Work out the finished part from the listing and answer in its coordinate system (mm). A direction names the side the tool comes from. Coordinates: 2 decimals unless noted, no trailing zeros. Order: outer loops, then holes, each group sorted by start corner. A loop starts at its lowest first (then second) coordinate and runs counter-clockwise, first axis right, second up.
1. Determine the mould class of faces 6 (the cylindrical face through (137.58, 20.95, -2.54)), 7 (the flat face through (-27.1, -18.5, 9.9)), 8 (the cylindrical face through (-1.302, -18.451, 27.915)), 9 (the cylindrical face through (-171.285, -22.813, 4.374)) for opening direction X: +X half, -X half, draft (parallel to the pull), parting line (faces both ways), or undercut.
2. The part is cut by section B-B, the plane z = 15. Give the vertices of the cut face in (x, y), then the cut area to 3 significant figures.
3. A tool of negligible diameter and unlimited length cuts with its end or side. For faces 1 (the flat face through (-7, -22, 9)), 2 (the flat face through (5, 0, 0)), 3 (the cylindrical face through (-174.519, -0.35, 6.433)), 4 (the flat face through (-7, -15, 9)), 5 (the flat face through (7, 22, 9)), from which of +Z, -Z, +X, -X, +Y, -Y can it reach the whole face along a straight path? Write none if from no direction.
4. Flat-ended cylindrical pins translate along their axes: pin 1 Ø12 at (y, z) = (-1, 21.5) entering from +X; pin 2 Ø17.5 at (x, z) = (-5.5, 17.5) entering from +Y; pin 3 Ø5 at (y, z) = (8, 27) entering from -X. Find the tip coordinate at first contact, or state that the pin passes through.
5. The part is cut by section D-D, the plane x = 49. Give the vertices of the cut face in (y, z).
6. Find the intervals of material crossed by probe 1 along Y at (x, z) = (1, 6); probe 2 along Z at (x, y) = (0, -20); probe 3 along Z at (x, y) = (-79, 17.5), in increasing order.
7. The part is cut by section C-C, the plane y = 8.5. Give the vertices of the cut face in (x, z), then the cut area to 3 significant figures.
8. The part is cut by section A-A, the plane x = 0. Give the vertices of the cut face in (y, z).
```python
from build123d import *

# Parameters (mm, degrees)
F0_R     = 10
F1_DEPTH = 25
F2_W     = 30
F2_H     = 40.766016
F2_W_2   = 3
F3_DEPTH = 40
F5_DEPTH = 40.001


with BuildPart() as f1:
    # F0 (on Front) → F1 (new body, symmetric)
    with BuildSketch(Plane.XZ):
        with BuildLine():
            Line((-31.201941, 0), (-147.458184, 0))
            ThreePointArc((-147.458184, 0), (-174.873856, 6.613726), (-196.258555, 25))
            Line((-196.258555, 25), (-197.63568, 23.332754))
            ThreePointArc((-197.63568, 23.332754), (-175.850829, 3.315154), (-147.458184, -5))
            Line((-147.458184, -5), (153.741445, -5))
            Line((153.741445, -5), (153.741445, 0))
            Line((153.741445, 0), (31.201941, 0))
            Line((31.201941, 0), (-31.201941, 0))
        make_face()
        with BuildLine():
            Line((-23.096988, 19.567086), (-31.201941, 0))
            Line((-31.201941, 0), (31.201941, 0))
            Line((31.201941, 0), (23.096988, 19.567086))
            ThreePointArc((23.096988, 19.567086), (0, 35), (-23.096988, 19.567086))
        make_face()
        with Locations((0, 18)):
            Circle(F0_R, mode=Mode.SUBTRACT)
    extrude(amount=F1_DEPTH, both=True)

    # F2 (on Right) → F3 (cut, symmetric)
    with BuildSketch(Plane.YZ):
        with Locations((0, 20.383008)):
            Rectangle(F2_W, F2_H)
        with Locations((-23.5, 20.383008)):
            Rectangle(F2_W_2, F2_H)
        with Locations((23.5, 20.383008)):
            Rectangle(F2_W_2, F2_H)
    extrude(amount=F3_DEPTH, both=True, mode=Mode.SUBTRACT)

    # F4 (on face) → F5 (cut, through all)
    with BuildSketch(Plane(origin=(0, 0, -5), x_dir=(1, 0, 0), z_dir=(0, 0, -1))):
        with BuildLine():
            ThreePointArc((-197.63568, 15), (-173.040312, 22.475658), (-147.458184, 25))
            Line((-147.458184, 25), (-197.63568, 25))
            Line((-197.63568, 25), (-197.63568, 15))
        make_face()
        with BuildLine():
            ThreePointArc((-147.458184, -25), (-173.040312, -22.475658), (-197.63568, -15))
            Line((-197.63568, -15), (-197.63568, -25))
            Line((-197.63568, -25), (-147.458184, -25))
        make_face()
        with BuildLine():
            ThreePointArc((153.741445, -14.029152), (137.337425, -21.027169), (119.951203, -25))
            Line((119.951203, -25), (153.741445, -25))
            Line((153.741445, -25), (153.741445, -14.029152))
        make_face()
        with BuildLine():
            Line((153.741445, 14.029152), (153.741445, 25))
            Line((153.741445, 25), (119.951203, 25))
            ThreePointArc((119.951203, 25), (137.714508, 22.188584), (153.741445, 14.029152))
        make_face()
    extrude(amount=-F5_DEPTH, mode=Mode.SUBTRACT)


solid = f1.part
```
Geometry says:
1. face 6: +X half
1. face 7: undercut
1. face 8: undercut
1. face 9: -X half
2. outline: (-190.88, -17.59) arc R130.89 ccw to (-187.19, -18.82) - (-187.19, 18.82) arc R130.89 ccw to (-190.88, 17.59) - close; (-24.99, -22) - (-9.54, -22) - (-9.54, -15) - (-24.99, -15) - close; (-24.99, 15) - (-9.54, 15) - (-9.54, 22) - (-24.99, 22) - close; (9.54, -22) - (24.99, -22) - (24.99, -15) - (9.54, -15) - close; (9.54, 15) - (24.99, 15) - (24.99, 22) - (9.54, 22) - close
2. area: 567 mm2
3. face 1: +Z, +X, -Y
3. face 2: +Z
3. face 3: +Z, +Y, -Y
3. face 4: +Z, +X
3. face 5: +Z, +X, +Y
4. pin 1: stops at x = -187.75
4. pin 2: stops at y = 22
4. pin 3: stops at x = -196.67
5. outline: (-25, -5) - (25, -5) - (25, 0) - (-25, 0) - close
6. probe 1: y = -22 to -15, 15 to 22
6. probe 2: z = -5 to 8, 28 to 35
6. probe 3: z = -5 to 0
7. outline: (-197.64, 23.33) arc R65.13 ccw to (-147.46, -5) - (153.74, -5) - (153.74, 0) - (-147.46, 0) arc R60.13 cw to (-196.26, 25) - close
7. area: 1,710 mm2
8. outline: (-25, -5) - (25, -5) - (25, 0) - (22, 0) - (22, 8) - (15, 8) - (15, 0) - (-15, 0) - (-15, 8) - (-22, 8) - (-22, 0) - (-25, 0) - close; (-22, 28) - (-15, 28) - (-15, 35) - (-22, 35) - close; (15, 28) - (22, 28) - (22, 35) - (15, 35) - close
